CAD build for the part. Positions are in the model's coordinates, mm. Round coordinates to 2 decimals unless told otherwise and drop trailing zeros. Loops run counter-clockwise (first coordinate to the right, second up) from the corner with the lowest first, then second, coordinate; pieces in that order, holes last. Notation, with made-up numbers: M 56.25,80 L 60.25,80 A20 cw 60.25,106 Z; hole C -12,-15 d4. An arc over 180 degrees is marked long. Use a Markdown table: item, result. Add a question column.
(1) Flat gauge pins, fed straight in: P1, Ø0.9, axis at x = 2, y = -23.5, coming from the +Z side; P2, Ø10, axis at x = 16.5, z = -13, coming from the -Y side; P3, Ø10, axis at x = 17.5, z = -9.5, coming from the +Y side; P4, Ø5, axis at y = -18.5, z = 18.5, coming from the -X side. Where does each tip first touch, or does it go through?
(2) Wall check: L1, parallel to Z at x = 2.5, y = 19; L2, parallel to Z at x = 17, y = 1.5; L3, parallel to Y at x = 2.5, z = -12.5. Give the ranges that are in metal, low to high.
(3) Band-saw the part on A-A, the plane x = 7.5. Write the cut outline in (y, z), and give its area (3 significant figures).
(4) Band-saw the part on C-C, the plane y = 6. Write the cut outline in (x, z).
(5) Band-saw the part on B-B, the plane z = 15. Write the cut outline in (x, y), and give its area (3 significant figures).
Autodesk Inventor part; units mm, degrees
ref_plane "Work Plane1" through (0, -24, 0) normal (0, 1, 0) x (-1, 0, 0)
ref_plane "Work Plane2" through (0, 24, 0) normal (0, 1, 0) x (-1, 0, 0)
ref_plane "Work Plane3" through (0, 0, 24) normal (0, 0, 1) x (1, 0, 0)
sketch "Sketch1" plane through (0, 0, 0) normal (0, 0, 1) x (1, 0, 0)
  line L0 (0, 0) -> (0, 22.5)
  line L1 (0, 22.5) -> (0, 0)
  line L2 (22.5, 0) -> (0, 0)
  arc A0 (22.5, 0) -> (0, 22.5) centre (0, 0) ccw
  dimension "d3" = 22.5
  dimension "d4" = 22.5
revolve "Revolution2" add sketch "Sketch1" angle 360 about axis through (22.5, 0, 0) along (-1, 0, 0)
shell "Shell1" thickness 1.5 removed faces 1 at (0, 7.2821, 1.7949)
ref_plane "Work Plane1" through (0, -24, 0) normal (0, 1, 0) x (-1, 0, 0)
ref_plane "Work Plane2" through (0, 24, 0) normal (0, 1, 0) x (-1, 0, 0)
ref_plane "Work Plane3" through (0, 0, 24) normal (0, 0, 1) x (1, 0, 0)
ref_plane "Work Plane4" through (0, 0, -24) normal (0, 0, 1) x (1, 0, 0)
sketch "Sketch2" plane through (0, 0, 24) normal (0, 0, 1) x (1, 0, 0)
  line L0 (0, -22.5) -> (0, 22.5)
  line L1 (0, -1.5) -> (3, -1.5)
  line L2 (3, -1.5) -> (3, 1.5)
  line L3 (3, 1.5) -> (0, 1.5)
  line L4 (0, 1.5) -> (0, -1.5)
  point P0 (0, 0)
  dimension "d24" = 3
  dimension "d25" = 3
sketch "Sketch3" plane through (0, -24, 0) normal (0, 1, 0) x (-1, 0, 0)
  line L0 (0, 22.5) -> (0, -22.5)
  line L1 (0, -1.5) -> (-3, -1.5)
  line L2 (-3, -1.5) -> (-3, 1.5)
  line L3 (-3, 1.5) -> (0, 1.5)
  line L4 (0, 1.5) -> (0, -1.5)
  point P0 (0, 0)
  dimension "d26" = 3
  dimension "d27" = 3
sketch "Sketch4" plane through (0, 0, -24) normal (0, 0, 1) x (1, 0, 0)
  line L0 (0, -22.5) -> (0, 22.5)
  line L1 (0, -1.5) -> (3, -1.5)
  line L2 (3, -1.5) -> (3, 1.5)
  line L3 (3, 1.5) -> (0, 1.5)
  line L4 (0, 1.5) -> (0, -1.5)
  point P0 (0, 0)
  dimension "d28" = 3
  dimension "d29" = 3
sketch "Sketch5" plane through (0, 24, 0) normal (0, 1, 0) x (-1, 0, 0)
  line L0 (0, -1.4364) -> (-3, -1.4364)
  line L1 (-3, -1.4364) -> (-3, 1.5636)
  line L2 (-3, 1.5636) -> (0, 1.5636)
  line L3 (0, 1.5636) -> (0, -1.4364)
  point P0 (0, 0)
  dimension "d30" = 3
  dimension "d31" = 3
extrude "Extrusion5" add sketch "Sketch2" against normal up to next
extrude "Extrusion6" add sketch "Sketch3" along normal up to next
extrude "Extrusion7" add sketch "Sketch4" along normal up to next
extrude "Extrusion8" add sketch "Sketch5" against normal up to next
properties part number "Liner 2" material "Polyethylene, High Density"
Return value:
| question | item | result |
|---|---|---|
| 1 | P1 | z = 1.5 |
| 1 | P2 | y = -15.81 |
| 1 | P3 | y = 16.85 |
| 1 | P4 | through |
| 2 | L1 | -11.79 to -8.59, 8.59 to 11.79 |
| 2 | L2 | -14.66 to -12.24, 12.24 to 14.66 |
| 2 | L3 | -18.54 to -16.69, 16.69 to 18.54 |
| 3 | outline | C 0,0 d42.43; hole C 0,0 d39.23 |
| 3 | area | 205 mm^2 |
| 4 | outline | M 0,-21.69 A21.69 ccw 0,21.69 L 0,20.12 A20.12 cw 0,-20.12 Z |
| 5 | outline | M 0,-16.77 A16.77 ccw 0,16.77 L 0,14.7 A14.7 cw 0,-14.7 Z |
| 5 | area | 102 mm^2 |
